Build history of the part. All positions in model axes, mm. Face numbers are marked on the shaded views. A direction names the side the tool comes from. Round coordinates to 2 decimals unless told otherwise and drop trailing zeros. Loops run counter-clockwise (first coordinate to the right, second up) from the corner with the lowest first, then second, coordinate; pieces in that order, holes last. Notation, with made-up numbers: (77, 39.5) - (119, 39.5) arc R12 cw to (119, 50.5) - close; hole circle Ø5 at (-39, 86.25). An arc over 180 degrees is marked (long way). Use a Markdown table: item, result.
from build123d import *

# Parameters (mm, degrees)
F0_W      = 195.9098130465
F0_H      = 83.3830982447
F1_DEPTH  = 4.7625
F2_W      = 195.9098130465
F2_H      = 3.2381750643
F3_DEPTH  = 34.8488
F4_R      = 3.6792614691
F5_DEPTH  = 3.175
F6_W      = 195.9098130465
F6_H      = 4.0477178991
F7_DEPTH  = 49.53
F8_R      = 5.08
F9_DEPTH  = 317.5
F10_DEPTH = 317.5
F11_DEPTH = 123.3551
F12_DEPTH = 123.3551


with BuildPart() as f1:
    # F0 (on Right) → F1 (new body)
    with BuildSketch(Plane.YZ):
        Rectangle(F0_W, F0_H)
    extrude(amount=F1_DEPTH)

    # F2 (on face) → F3 (join)
    with BuildSketch(Plane.YZ.offset(4.7625)):
        with Locations((0, -40.0724615902)):
            Rectangle(F2_W, F2_H)
    extrude(amount=F3_DEPTH)

    # F4
    f4_edges = [f1.edges().sort_by_distance(p)[0] for p in [
        (0, 0, -41.691549),
    ]]
    fillet(f4_edges, radius=F4_R)

    # F5 (cut): a face of the model
    f5_faces = [f1.faces().sort_by_distance(p)[0] for p in [
        (39.6113, 0, -40.0724615902),
    ]]
    extrude(f5_faces, amount=-F5_DEPTH, mode=Mode.SUBTRACT)

    # F6 (on face) → F7 (join)
    with BuildSketch(Plane.YZ.offset(4.7625)):
        with Locations((0, 39.6676901728)):
            Rectangle(F6_W, F6_H)
    extrude(amount=F7_DEPTH)

    # F8
    f8_edges = [f1.edges().sort_by_distance(p)[0] for p in [
        (0, 0, 41.691549),
    ]]
    fillet(f8_edges, radius=F8_R)

    # F9 (add): a face of the model
    f9_faces = [f1.faces().sort_by_distance(p)[0] for p in [
        (29.68625, 97.9549065232, 40.696540749),
    ]]
    extrude(f9_faces, amount=F9_DEPTH)

    # F10 (add): a face of the model
    f10_faces = [f1.faces().sort_by_distance(p)[0] for p in [
        (0.9950083733, -97.9549065232, -0.7003692655),
    ]]
    extrude(f10_faces, amount=F10_DEPTH)

    # F11 (cut): a face of the model
    f11_faces = [f1.faces().sort_by_distance(p)[0] for p in [
        (29.68625, 415.4549065232, 40.696540749),
    ]]
    extrude(f11_faces, amount=-F11_DEPTH, mode=Mode.SUBTRACT)

    # F12 (cut): a face of the model
    f12_faces = [f1.faces().sort_by_distance(p)[0] for p in [
        (0.9950083733, -415.4549065232, -0.7003692655),
    ]]
    extrude(f12_faces, amount=-F12_DEPTH, mode=Mode.SUBTRACT)


solid = f1.part
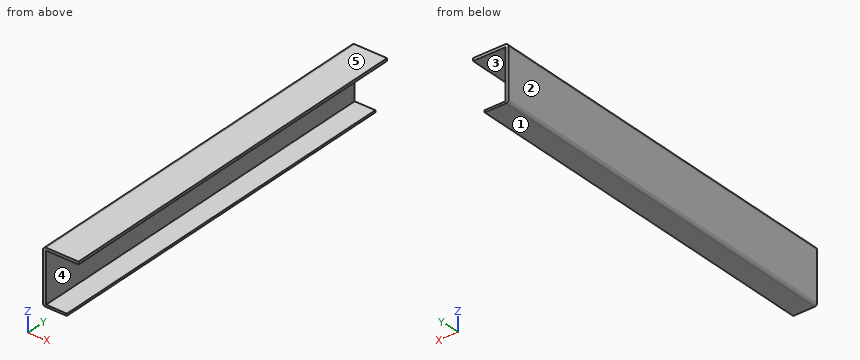
Q1. Probe line 1 (Z direction, x = 32, y = -78); line 2 (X direction, y = 170, z = -8); line 3 (Z direction, x = 38, y = 2). List the from-to ranges inside material, lowest first.
Results found:
| item | result |
|---|---|
| line 1 | z = -41.69 to -38.45, 37.64 to 41.69 |
| line 2 | x = 0 to 4.76 |
| line 3 | z = 37.64 to 41.69 |
Q2. Cut at D-D, the plane x = 44. List the corners of the cut face in (y, z).
Results found:
| item | result |
|---|---|
| outline | (-292.1, 37.64) - (292.1, 37.64) - (292.1, 41.69) - (-292.1, 41.69) - close |
Q3. Cut at B-B, the plane y = 125.5. List the corners of the cut face in (x, z), plus the area to 3 significant figures.
Results found:
| item | result |
|---|---|
| outline | (0, -38.01) arc R3.68 ccw to (3.68, -41.69) - (36.44, -41.69) - (36.44, -38.45) - (4.76, -38.45) - (4.76, 37.64) - (54.29, 37.64) - (54.29, 41.69) - (5.08, 41.69) arc R5.08 ccw to (0, 36.61) - close |
| area | 692 mm2 |
Q4. Pull direction Z, two halves, no side cores. Call the marked faces 1, 2 and 3: pulls with the +Z half, pulls with the -Z half, needs draft (parallel to the pull), parting line crosses it, or undercut.
Results found:
| item | result |
|---|---|
| face 1 | pulls with the -Z half |
| face 2 | needs draft |
| face 3 | undercut |
Q5. Drop flat-ended pins along their axis: pin 1 (2.5 mm diameter, centred on y = -55, z = -39.5, fed in from +X); pin 2 (8 mm diameter, centred on y = -99, z = -4.5, fed in from +X). Give the stop position or say it passes through.
Results found:
| item | result |
|---|---|
| pin 1 | stops at x = 36.44 |
| pin 2 | stops at x = 4.76 |
Q6. Cut at C-C, the plane z = 29.5. List the corners of the cut face in (x, y), plus the area to 3 significant figures.
Results found:
| item | result |
|---|---|
| outline | (0, -292.1) - (4.76, -292.1) - (4.76, 292.1) - (0, 292.1) - close |
| area | 2,780 mm2 |
Q7. Cut at A-A, the plane x = 22.5. List the corners of the cut face in (y, z), plus the area to 3 significant figures.
Results found:
| item | result |
|---|---|
| outline | (-292.1, -41.69) - (292.1, -41.69) - (292.1, -38.45) - (-292.1, -38.45) - close; (-292.1, 37.64) - (292.1, 37.64) - (292.1, 41.69) - (-292.1, 41.69) - close |
| area | 4,260 mm2 |
Q8. Which spindle directions (+Z, -Z, +X, -X, +Y, -Y) get a long thin tool onto all of the face, cutting with end or side? Do the marked faces 4 and 5. Say none if no direction does.
Results found:
| item | result |
|---|---|
| face 4 | +X, +Y, -Y |
| face 5 | +Z, +X, -X, +Y, -Y |
